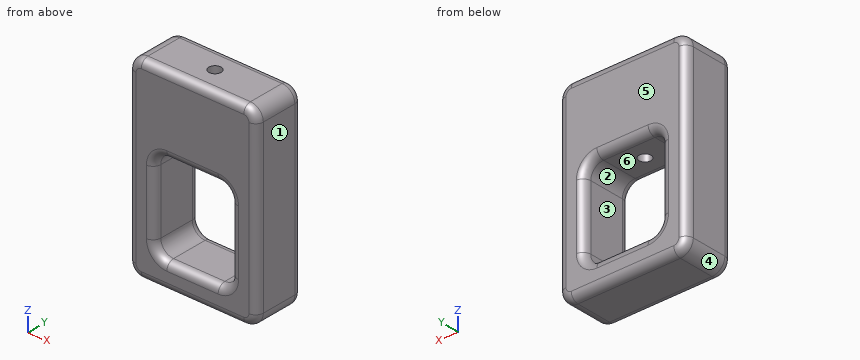
```python
from build123d import *

# Parameters (mm, degrees)
SKETCH1_W           = 12.7
SKETCH1_H           = 19.05
BOSS_EXTRUDE1_DEPTH = 5.08
SKETCH2_W           = 7.62
SKETCH2_H           = 8.89
CUT_EXTRUDE1_DEPTH  = 13.524157656
SKETCH3_R           = 0.5999988
CUT_EXTRUDE3_DEPTH  = 7.62
FILLET1_R           = 1.27
FILLET2_R           = 1.27
FILLET3_R           = 0.762
FILLET4_R           = 0.762


with BuildPart() as part:
    # Sketch1 → Boss-Extrude1 (new body)
    with BuildSketch(Plane(origin=(0, 0, 0), x_dir=(1, 0, 0), z_dir=(0, 1, 0))):
        Rectangle(SKETCH1_W, SKETCH1_H)
    extrude(amount=BOSS_EXTRUDE1_DEPTH)

    # Sketch2 → Cut-Extrude1 (cut, through all)
    with BuildSketch(Plane.XZ):
        with Locations((0, -2.54)):
            Rectangle(SKETCH2_W, SKETCH2_H)
    extrude(amount=-CUT_EXTRUDE1_DEPTH, mode=Mode.SUBTRACT)

    # Sketch3 → Cut-Extrude3 (cut)
    with BuildSketch(Plane.XY.offset(9.525)):
        with Locations((0, 2.54)):
            Circle(SKETCH3_R)
    extrude(amount=-CUT_EXTRUDE3_DEPTH, mode=Mode.SUBTRACT)

    # Fillet1
    fillet1_edges = [part.edges().sort_by_distance(p)[0] for p in [
        (6.35, 2.54, 9.525),
        (-6.35, 2.54, 9.525),
        (-6.35, 2.54, -9.525),
        (6.35, 2.54, -9.525),
    ]]
    fillet(fillet1_edges, radius=FILLET1_R)

    # Fillet2
    fillet2_edges = [part.edges().sort_by_distance(p)[0] for p in [
        (3.81, 2.54, 1.905),
        (3.81, 2.54, -6.985),
        (-3.81, 2.54, -6.985),
        (-3.81, 2.54, 1.905),
    ]]
    fillet(fillet2_edges, radius=FILLET2_R)

    # Fillet3
    fillet3_edges = [part.edges().sort_by_distance(p)[0] for p in [
        (0, 5.08, -9.525),
        (6.35, 5.08, 0),
        (-6.35, 5.08, 0),
        (0, 5.08, 9.525),
        (5.978025612, 5.08, 9.153025612),
        (-5.978025612, 5.08, 9.153025612),
        (-5.978025612, 5.08, -9.153025612),
        (5.978025612, 5.08, -9.153025612),
    ]]
    fillet(fillet3_edges, radius=FILLET3_R)

    # Fillet4
    fillet4_edges = [part.edges().sort_by_distance(p)[0] for p in [
        (0, 0, -9.525),
        (6.35, 0, 0),
        (0, 0, 9.525),
        (-6.35, 0, 0),
        (5.978025612, 0, 9.153025612),
        (-5.978025612, 0, 9.153025612),
        (-5.978025612, 0, -9.153025612),
        (5.978025612, 0, -9.153025612),
        (0, 0, -6.985),
        (0, 5.08, -6.985),
        (-3.81, 0, -2.54),
        (-3.81, 5.08, -2.54),
        (3.81, 0, -2.54),
        (3.81, 5.08, -2.54),
        (0, 0, 1.905),
        (0, 5.08, 1.905),
        (-3.438025612, 0, -6.613025612),
        (-3.438025612, 5.08, -6.613025612),
        (3.438025612, 0, -6.613025612),
        (3.438025612, 5.08, -6.613025612),
        (-3.438025612, 0, 1.533025612),
        (-3.438025612, 5.08, 1.533025612),
        (3.438025612, 0, 1.533025612),
        (3.438025612, 5.08, 1.533025612),
    ]]
    fillet(fillet4_edges, radius=FILLET4_R)


solid = part.part
```
The model under review builds one solid part; all positions refer to its coordinate system, in mm. Face numbers are marked on the shaded views. A direction names the side the tool comes from. Round coordinates to 2 decimals unless told otherwise and drop trailing zeros. Write each loop counter-clockwise with the first axis right and the second up, starting at its lowest first coordinate (ties: lowest second). Pieces come first, ordered by that corner, then holes. Notation, with made-up numbers: (64.25, 27.5) - (112.25, 27.5) arc R24 ccw to (112.25, 59.5) - close; hole circle Ø4 at (14, -29.75). An arc over 180 degrees is marked (long way). Answer as CSV lines item,"result". Start each with the question number.
(1) For the marked faces 5 and 6, list the 3-axis set-ups (+Z, -Z, +X, -X, +Y, -Y) from which the entire face can be reached by the end or side of a thin tool; tool diameter is ignored.
(2) We need section A-A on z = -2.75. State the section outline as (x, y) points, plus the area to 3 significant figures.
(3) We need section B-B on x = 0. State the section outline as (y, z) points (3 decimals), plus the area to 3 significant figures.
(4) For pin 1 Ø1 at (x, y) = (0, 2.54) entering from +Z (3 decimals); pin 2 Ø1.5 at (x, z) = (3.5, -3.5) entering from -Y, all flat-tipped, find the tip position at first contact; note any pin that passes through.
(5) To check wall thickness, follow line 1 (Z direction, x = -1, y = 1.4) (3 decimals); line 2 (Y direction, x = 0, z = 6.75); line 3 (X direction, y = 1.4, z = -3.75). State the ranges of each line that lie inside material, in increasing order.
(6) We need section D-D on z = 5.25. State the section outline as (x, y) points.
(7) We need section C-C on y = 1. State the section outline as (x, z) points (3 decimals), plus the area to 3 significant figures.
(8) Draft analysis for pull direction X (two halves, no side actions). For the marked faces 1, 2, 3 and 4, state which applies: pulls with the +X half, pulls with the -X half, needs draft (parallel to the pull), parting line crosses it, or undercut.
Worked answers:
1,face 5,"+Z, -Z, +X, -X, +Y"
1,face 6,"+Y, -Y"
2,outline,"(-6.35, 0.76) arc R0.76 ccw to (-5.59, 0) - (-4.57, 0) arc R0.76 ccw to (-3.81, 0.76) - (-3.81, 4.32) arc R0.76 ccw to (-4.57, 5.08) - (-5.59, 5.08) arc R0.76 ccw to (-6.35, 4.32) - close; (3.81, 0.76) arc R0.76 ccw to (4.57, 0) - (5.59, 0) arc R0.76 ccw to (6.35, 0.76) - (6.35, 4.32) arc R0.76 ccw to (5.59, 5.08) - (4.57, 5.08) arc R0.76 ccw to (3.81, 4.32) - close"
2,area,"24.8 mm²"
3,outline,"(0, -8.763) arc R0.762 ccw to (0.762, -9.525) - (4.318, -9.525) arc R0.762 ccw to (5.08, -8.763) - (5.08, -7.747) arc R0.762 ccw to (4.318, -6.985) - (0.762, -6.985) arc R0.762 ccw to (0, -7.747) - close; (0, 2.667) arc R0.762 ccw to (0.762, 1.905) - (1.94, 1.905) - (1.94, 9.525) - (0.762, 9.525) arc R0.762 ccw to (0, 8.763) - close; (3.14, 1.905) - (4.318, 1.905) arc R0.762 ccw to (5.08, 2.667) - (5.08, 8.763) arc R0.762 ccw to (4.318, 9.525) - (3.14, 9.525) - close"
3,area,"41.5 mm²"
4,pin 1,"z = -6.985"
4,pin 2,"y = 0.07"
5,line 1,"-9.525 to -6.985, 1.905 to 9.525"
5,line 2,"0 to 1.94, 3.14 to 5.08"
5,line 3,"-6.35 to -3.81, 3.81 to 6.35"
6,outline,"(-6.35, 0.76) arc R0.76 ccw to (-5.59, 0) - (5.59, 0) arc R0.76 ccw to (6.35, 0.76) - (6.35, 4.32) arc R0.76 ccw to (5.59, 5.08) - (-5.59, 5.08) arc R0.76 ccw to (-6.35, 4.32) - close; hole circle Ø1.2 at (0, 2.54)"
7,outline,"(-6.35, -8.255) arc R1.27 ccw to (-5.08, -9.525) - (5.08, -9.525) arc R1.27 ccw to (6.35, -8.255) - (6.35, 8.255) arc R1.27 ccw to (5.08, 9.525) - (-5.08, 9.525) arc R1.27 ccw to (-6.35, 8.255) - close; hole (-3.81, -5.715) arc R1.27 ccw to (-2.54, -6.985) - (2.54, -6.985) arc R1.27 ccw to (3.81, -5.715) - (3.81, 0.635) arc R1.27 ccw to (2.54, 1.905) - (-2.54, 1.905) arc R1.27 ccw to (-3.81, 0.635) - close"
7,area,"174 mm²"
8,face 1,"pulls with the +X half"
8,face 2,"undercut"
8,face 3,"undercut"
8,face 4,"pulls with the -X half"
